Source: CAD feature listing. Evaluate the final solid. Frame: model axes, mm. Face numbers are marked on the shaded views. A direction names the side the tool comes from. Coordinates: 2 decimals unless noted, no trailing zeros. Write each loop counter-clockwise with the first axis right and the second up, starting at its lowest first coordinate (ties: lowest second). Pieces come first, ordered by that corner, then holes. Notation, with made-up numbers: (78.5, -36.75) -> (129.5, -36.75) arc R23 cw to (129.5, -2.75) -> close; hole circle Ø9 at (40.25, 46). An arc over 180 degrees is marked (long way). One line per item, written item: value. Start each with the question number.
1. Line query: line 1 (Y direction, x = 3.25, z = 1.5); line 2 (X direction, y = 6, z = 3.5); line 3 (Y direction, x = -4, z = 2.25). Output: solid intervals per line, ascending.
2. Section query B-B, the plane x = -0.5. Output: boundary loops of the cut face in (y, z), and give its area (3 significant figures).
3. First-contact query: P1, Ø2, axis at x = -7.5, y = 7.5, coming from the -Z side; P2, Ø5, axis at x = -4, y = 6, coming from the +Z side; P3, Ø0.5, axis at y = 10.5, z = 4.5, coming from the +X side. Flat tips, straight axial feed; report the tip coordinate or a pass-through.
4. Mould query, pull axis Y, two halves, no side actions, for the marked faces 1, 2 and 3. Classes: released by +Y, released by -Y, zero draft, split by the parting line, or undercut.
5. Section query A-A, the plane x = 1.75. Output: boundary loops of the cut face in (y, z), and give its area (3 significant figures).
6. Section query C-C, the plane y = 6. Output: boundary loops of the cut face in (x, z).
7. Access query for the marked faces 4 and 5. Directions: +Z, -Z, +X, -X, +Y, -Y. A direction counts if a zero-diameter tool reaches every point of the face in a straight line with its end or side. Return the directions, or none.
Autodesk Inventor part; units mm, degrees
ref_plane "YZ Plane" through (0, 0, 0) normal (1, 0, 0) x (0, 1, 0)
ref_plane "XZ Plane" through (0, 0, 0) normal (0, 1, 0) x (-1, 0, 0)
ref_plane "XY Plane" through (0, 0, 0) normal (0, 0, 1) x (1, 0, 0)
sketch "Sketch1" plane through (0, 0, 0) normal (0, 1, 0) x (-1, 0, 0)
  arc A0 (-10, 0) -> (10, 0) centre (0, 113.8115) ccw
  line L0 (10, 0) -> (-10, 0) construction
  line L1 (10, 0) -> (-10, 0)
  line L2 (-10, 0) -> (-10, 6)
  line L3 (-10, 6) -> (10, 6)
  line L4 (10, 6) -> (10, 0)
  point P0 (0, 0)
  point P1 (0, 0)
  dimension "d0" = 114.25
  dimension "d1" = 20
  dimension "d2" = 6
extrude "Extrusion1" add sketch "Sketch1" along normal blind 12
sketch "Sketch2" plane through (-10, 0, 6) normal (0, 0, 1) x (1, 0, 0)
  line L0 (20, 0) -> (0, 0) construction
  line L1 (20, 0) -> (20, 12) construction
  line L2 (0, 12) -> (20, 12) construction
  line L3 (0, 0) -> (0, 12) construction
  circle A0 centre (6, 6) radius 4
  arc A1 (20, 1) -> (8.0951, 2.5925) centre (13.0714, -5.501) ccw
  line L4 (10, 6) -> (10, 0) construction
  line L5 (6, 10) -> (20, 10)
  line L6 (20, 1) -> (20, 0)
  line L7 (20, 0) -> (0, 0) construction
  line L8 (20, 0) -> (0, 0)
  line L9 (0, 0) -> (0, 12)
  line L10 (20, 12) -> (0, 12) construction
  line L11 (20, 12) -> (20, 10)
  line L12 (20, 12) -> (0, 12)
  line L13 (10.6891, 4) -> (16.5284, 4) construction
  arc A2 (20, 0) -> (6.1427, 0) centre (13.0714, -5.501) ccw
  line L14 (20, 1) -> (20, 10)
  point P0 (20, 6)
  dimension "d5" = 8
  dimension "d7" = 1
  dimension "d8" = 2
  dimension "d14" = 2
extrude "Extrusion2" cut sketch "Sketch2" against normal through all contours A0 | A0 L5 L14 A1 | L8 A2
fillet "Fillet1" radius 0.32 2 edges at (10, 0, 3) (10, 1, 3)
fillet "Fillet2" radius 2 4 edges at (-3.8573, 0, 2.8133) (-10, 12, 3) (-10, 0, 3) (10, 10, 3)
sketch "Sketch3" plane through (-8, 0, 6) normal (0, 0, 1) x (1, 0, 0)
  arc A0 (16, 10) -> (18, 12) centre (16, 12) ccw construction
  line L0 (0, 12) -> (18, 12) construction
  arc A1 (0, 12) -> (-2, 10) centre (0, 10) ccw construction
  line L1 (-2, 2) -> (-2, 10) construction
  arc A2 (-2, 2) -> (0, 0) centre (0, 2) ccw construction
  line L2 (3.2362, 0) -> (0, 0) construction
  arc A3 (3.2362, 0) -> (4.6809, 0.6169) centre (3.2362, 2) ccw construction
  arc A4 (17.4493, 0.63) -> (4.6809, 0.6169) centre (11.0714, -5.501) ccw construction
  arc A5 (17.4493, 0.63) -> (18, 0.8517) centre (17.68, 0.8517) ccw construction
  line L3 (18, 0.8517) -> (18, 0.8721) construction
  arc A6 (18, 0.8721) -> (17.9103, 1.0943) centre (17.68, 0.8721) ccw construction
  arc A7 (17.9103, 1.0943) -> (6.0951, 2.5925) centre (11.0714, -5.501) ccw construction
  arc A8 (4, 10) -> (6.0951, 2.5925) centre (4, 6) ccw construction
  line L4 (4, 10) -> (16, 10) construction
  line L5 (-2, 12) -> (18, 12)
  line L6 (18, 12) -> (18, 10.6)
  line L7 (18, 10.6) -> (-2, 10.6)
  line L8 (-2, 10.6) -> (-2, 12)
  line L9 (16, 10.6) -> (18, 10.6)
  line L10 (18, 10.6) -> (18, 10)
  line L11 (18, 10) -> (16, 10)
  line L12 (16, 10) -> (16, 10.6)
  point P0 (8, 0)
  dimension "d15" = 20
  dimension "d16" = 1.4
extrude "Extrusion3" cut sketch "Sketch3" against normal blind 10
properties part number "receiving_clip"
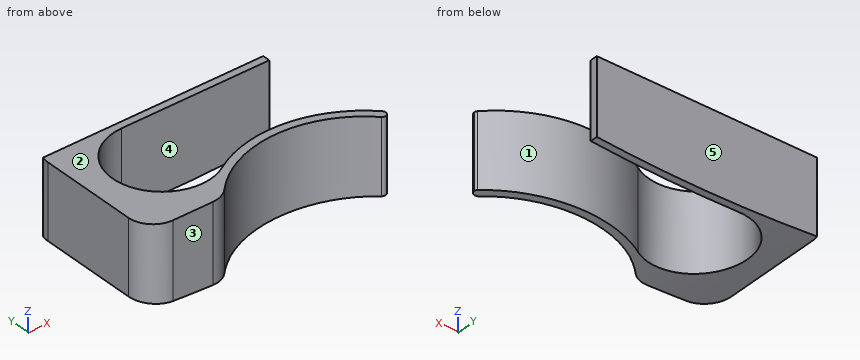
Computed values:
1. line 1: y = 3.34 to 4, 10 to 10.6
1. line 2: x = -10 to -8
1. line 3: y = 0.15 to 2, 10 to 10.6
2. outline: (2.59, -0.44) -> (3.3, -0.44) -> (3.3, 6) -> (2.59, 6) -> close; (10, -0.44) -> (10.6, -0.44) -> (10.6, 6) -> (10, 6) -> close
2. area: 8.43 mm²
3. P1: stops at z = -0.21
3. P2: passes through
3. P3: stops at x = 8
4. face 1: undercut
4. face 2: zero draft
4. face 3: released by -Y
5. outline: (3.25, -0.43) -> (3.91, -0.43) -> (3.91, 6) -> (3.25, 6) -> close; (10, -0.43) -> (10.6, -0.43) -> (10.6, 6) -> (10, 6) -> close
5. area: 8.10 mm²
6. outline: (-10, 0) arc R114.25 ccw to (-8, -0.16) -> (-8, 6) -> (-10, 6) -> close
7. face 4: +Z, -Z, +X
7. face 5: +Z, -Z, +X, -X, +Y
